from build123d import *

# Parameters (mm, degrees)
F1_DEPTH = 15
F2_R     = 5.6469971394
F3_DEPTH = 16
F4_R     = 5.9634440704
F5_DEPTH = 5
F6_R     = 1


with BuildPart() as f1:
    # F0 (on Front) → F1 (new body)
    with BuildSketch(Plane.XZ):
        with BuildLine():
            ThreePointArc((4.051797674, -14.4424006179), (11.9535970551, -9.0615405669), (15, 0))
            ThreePointArc((15, 0), (11.9535970551, 9.0615405669), (4.051797674, 14.4424006179))
            ThreePointArc((4.051797674, 14.4424006179), (-15, 0), (4.051797674, -14.4424006179))
        make_face()
        with BuildLine():
            ThreePointArc((4.051797674, 14.4424006179), (11.9535970551, 9.0615405669), (15, 0))
            ThreePointArc((15, 0), (11.9535970551, -9.0615405669), (4.051797674, -14.4424006179))
            Line((4.051797674, -14.4424006179), (38.3712039217, -4.8141335393))
            ThreePointArc((38.3712039217, -4.8141335393), (32.0206046971, 0), (38.3712039217, 4.8141335393))
            Line((38.3712039217, 4.8141335393), (4.051797674, 14.4424006179))
        make_face()
        with BuildLine():
            ThreePointArc((42.0206046971, 0), (41.0051370488, 3.0205135223), (38.3712039217, 4.8141335393))
            ThreePointArc((38.3712039217, 4.8141335393), (32.0206046971, 0), (38.3712039217, -4.8141335393))
            ThreePointArc((38.3712039217, -4.8141335393), (41.0051370488, -3.0205135223), (42.0206046971, 0))
        make_face()
    extrude(amount=F1_DEPTH)

    # F2 (on face) → F3 (cut)
    with BuildSketch(Plane.XZ.offset(15)):
        Circle(F2_R)
    extrude(amount=-F3_DEPTH, mode=Mode.SUBTRACT)

    # F4 (on face) → F5 (join)
    with BuildSketch(Plane(origin=(4.051797674, 0, 14.4424006179), x_dir=(0.9628267079, 0, -0.2701198449), z_dir=(0.2701198449, 0, 0.9628267079))):
        with Locations((20.6467304379, -7.5)):
            Circle(F4_R)
    extrude(amount=F5_DEPTH)

    # F6
    f6_edges = [f1.edges().sort_by_distance(p)[0] for p in [
        (19.539857, -7.5, 15.290287),
        (18.189258, -7.5, 10.476154),
    ]]
    fillet(f6_edges, radius=F6_R)


solid = f1.part
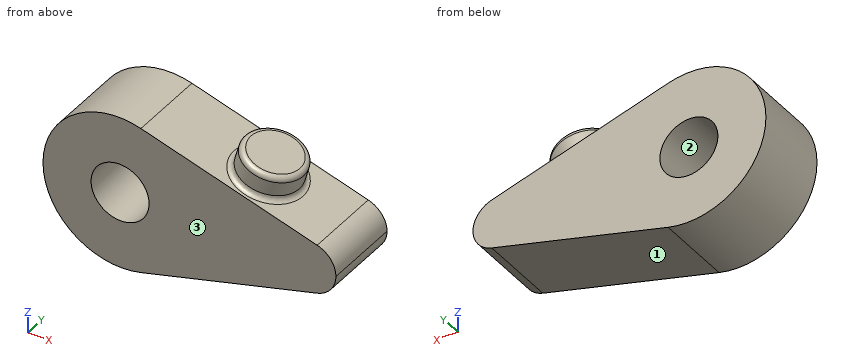
Geometry: final body of the model. Coordinates: model frame, mm. Face numbers are marked on the shaded views. Round coordinates to 2 decimals unless told otherwise and drop trailing zeros. Loops run counter-clockwise (first coordinate to the right, second up) from the corner with the lowest first, then second, coordinate; pieces in that order, holes last. Notation, with made-up numbers: M -24.5,0.25 L 24.5,0.25 A32 cw 24.5,36.25 Z; hole C 25,-39.75 d8. An arc over 180 degrees is marked long. Put each result on its own line as item: value. Start each with the question number.
(1) Section query A-A (x = 0). Return loops of the section in (y, z), then the cut area to 3 significant figures.
(2) Contact query for flat-ended pins moving along their axis: pin 1 Ø8 at (x, z) = (34.5, -9) entering from -Y; pin 2 Ø2 at (x, y) = (21, -11.5) entering from +Z; pin 3 Ø5 at (x, y) = (8, -10.5) entering from +Z; pin 4 Ø1 at (x, y) = (-7, -11.5) entering from +Z. Output: stop coordinate, or through.
(3) Draft query along X for the marked faces 1, 2 and 3. Return one class per face: +X half, -X half, draft (parallel to the pull), parting line (faces both ways), or undercut.
(4) Section query B-B (z = 1.5). Return loops of the section in (x, y).
(5) Section query C-C (z = -7). Return loops of the section in (x, y), then the cut area to 3 significant figures.
(6) Section query D-D (x = 36.5). Return loops of the section in (y, z).
(7) Material intervals for line 1 along Z through (x, y) = (0, -8.25); line 2 along Z through (x, y) = (-2, -5.5); line 3 along X through (y, z) = (-9.5, -4), sorted ascending. Write a range as [from, to].
Findings below:
1. outline: M -15,-15 L 0,-15 L 0,-5.65 L -15,-5.65 Z; M -15,5.65 L 0,5.65 L 0,15 L -15,15 Z
1. area: 281 mm2
2. pin 1: stops at y = -15
2. pin 2: stops at z = 14.8
2. pin 3: stops at z = 14.04
2. pin 4: stops at z = 13.52
3. face 1: +X half
3. face 2: undercut
3. face 3: draft
4. outline: M -14.92,-15 L -5.44,-15 L -5.44,0 L -14.92,0 Z; M 5.44,-15 L 41.79,-15 L 41.79,0 L 5.44,0 Z
5. outline: M -13.27,-15 L 30.58,-15 L 30.58,0 L -13.27,0 Z
5. area: 658 mm2
6. outline: M -15,-5.34 L 0,-5.34 L 0,5.34 L -15,5.34 Z
7. line 1: z = [-15, -5.65], [5.65, 15]
7. line 2: z = [-14.87, -5.28], [5.28, 14.87]
7. line 3: x = [-14.46, -3.99], [3.99, 40.02]
